```python
from build123d import *

# Parameters (mm, degrees)
BOSS_EXTRUDE1_DEPTH = 85
BOSS_EXTRUDE3_DEPTH = 2
SKETCH9_W           = 11.5
SKETCH9_H           = 2
BOSS_EXTRUDE8_DEPTH = 3
CHAMFER1_SIZE       = 3
SKETCH10_W          = 32
SKETCH10_H          = 85
BOSS_EXTRUDE9_DEPTH = 2
SKETCH11_W          = 15
SKETCH11_H          = 5
CUT_EXTRUDE1_DEPTH  = 108.588010242


with BuildPart() as part:
    # Sketch1 → Boss-Extrude1 (new body)
    with BuildSketch(Plane(origin=(0, 0, 0), x_dir=(1, 0, 0), z_dir=(0, 1, 0))):
        with BuildLine():
            Line((-29, -15), (-29, 15.762564303))
            ThreePointArc((-29, 15.762564303), (0, 25.341269657), (29, 15.762564303))
            Line((29, 15.762564303), (29, -15))
            Line((29, -15), (29, -17))
            Line((29, -17), (27.5, -17))
            Line((27.5, -17), (16, -17))
            Line((16, -17), (16, -15))
            Line((16, -15), (27.5, -15))
            Line((27.5, -15), (27.5, 15))
            ThreePointArc((27.5, 15), (0, 23.841269657), (-27.5, 15))
            Line((-27.5, 15), (-27.5, -15))
            Line((-27.5, -15), (-16, -15))
            Line((-16, -15), (-16, -17))
            Line((-16, -17), (-27.5, -17))
            Line((-27.5, -17), (-29, -17))
            Line((-29, -17), (-29, -15))
        make_face()
    extrude(amount=BOSS_EXTRUDE1_DEPTH)

    # Sketch3 → Boss-Extrude3 (add)
    with BuildSketch(Plane(origin=(0, 85, 0), x_dir=(1, 0, 0), z_dir=(0, 1, 0))):
        with BuildLine():
            Line((-16, -17), (16, -17))
            Line((16, -17), (29, -17))
            Line((29, -17), (29, 15.762564303))
            ThreePointArc((29, 15.762564303), (0, 25.341269657), (-29, 15.762564303))
            Line((-29, 15.762564303), (-29, -17))
            Line((-29, -17), (-16, -17))
        make_face()
    extrude(amount=BOSS_EXTRUDE3_DEPTH)

    # Sketch9 → Boss-Extrude8 (add)
    with BuildSketch(Plane(origin=(0, 0, 15), x_dir=(-1, 0, 0), z_dir=(0, 0, -1))):
        with Locations((-21.75, 15)):
            Rectangle(SKETCH9_W, SKETCH9_H)
        with Locations((21.75, 15)):
            Rectangle(SKETCH9_W, SKETCH9_H)
    extrude(amount=BOSS_EXTRUDE8_DEPTH)

    # Chamfer1
    chamfer1_edges = [part.edges().sort_by_distance(p)[0] for p in [
        (-21.75, 14, 15),
        (21.75, 14, 15),
    ]]
    chamfer(chamfer1_edges, length=CHAMFER1_SIZE - 0.0001)  # a hair under: the kernel refuses the full size

    # Sketch10 → Boss-Extrude9 (add)
    with BuildSketch(Plane.XY.offset(17)):
        with Locations((0, 42.5)):
            Rectangle(SKETCH10_W, SKETCH10_H)
    extrude(amount=-BOSS_EXTRUDE9_DEPTH)

    # Sketch11 → Cut-Extrude1 (cut, through all)
    with BuildSketch(Plane(origin=(29, 0, 0), x_dir=(0, 0, -1), z_dir=(1, 0, 0))):
        with Locations((0, 7.985525628)):
            Rectangle(SKETCH11_W, SKETCH11_H)
    extrude(amount=-CUT_EXTRUDE1_DEPTH, mode=Mode.SUBTRACT)


solid = part.part
```
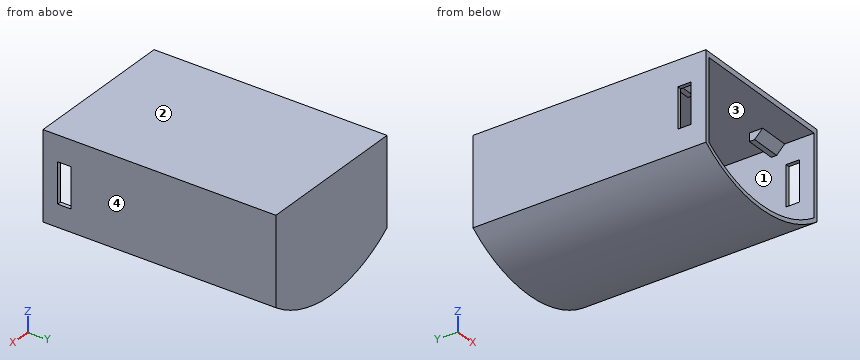
Work out the finished part from the listing and answer in its coordinate system (mm). Face numbers are marked on the shaded views. Round coordinates to 2 decimals unless told otherwise and drop trailing zeros. Write each loop counter-clockwise with the first axis right and the second up, starting at its lowest first coordinate (ties: lowest second). Pieces come first, ordered by that corner, then holes. Notation, with made-up numbers: (0, -2) -> (56, -2) arc R13 ccw to (56, 6) -> close; hole circle Ø3 at (-37.75, 48). An arc over 180 degrees is marked (long way). Write each question's results on one line, items separated by ' | '.
1) Consider line 1 along X through (y, z) = (70.5, 0); line 2 along Y through (x, z) = (-3, -7.5); line 3 along Z through (x, y) = (23, 14). Determine where each line is inside the solid, lowest interval first. Write a range as [from, to].
Findings:
line 1: x = [-29, -27.5], [27.5, 29] | line 2: y = [85, 87] | line 3: z = [-19.57, -17.86], [12, 17]
2) The part is cut by section D-D (z = -11). Write down the section's boundary in (x, y), and give its area (3 significant figures).
Findings:
outline: (-29, 0) -> (-27.5, 0) -> (-27.5, 85) -> (27.5, 85) -> (27.5, 0) -> (29, 0) -> (29, 87) -> (-29, 87) -> close | area: 371 mm²
3) Flat-ended cylindrical pins translate along their axes: pin 1 (1.2 mm diameter, centred on x = 28, y = 7, fed in from -Z); pin 2 (5 mm diameter, centred on x = -5, y = 66, fed in from -Z); pin 3 (8 mm diameter, centred on x = 23, y = 40, fed in from -Z). Find the tip coordinate at first contact, or state that the pin passes through.
Findings:
pin 1: stops at z = -16.9 | pin 2: stops at z = -25.28 | pin 3: stops at z = -21.48
4) The part is cut by section A-A (z = 3.5). Write down the section's boundary in (x, y), and give its area (3 significant figures).
Findings:
outline: (-29, 0) -> (-27.5, 0) -> (-27.5, 5.49) -> (-29, 5.49) -> close; (-29, 10.49) -> (-27.5, 10.49) -> (-27.5, 85) -> (27.5, 85) -> (27.5, 10.49) -> (29, 10.49) -> (29, 87) -> (-29, 87) -> close; (27.5, 0) -> (29, 0) -> (29, 5.49) -> (27.5, 5.49) -> close | area: 356 mm²
5) The part is cut by section B-B (y = 32). Write down the section's boundary in (x, z), and give its area (3 significant figures).
Findings:
outline: (-29, -15.76) arc R48.69 ccw to (29, -15.76) -> (29, 17) -> (-29, 17) -> close; hole (-27.5, -15) arc R47.19 ccw to (27.5, -15) -> (27.5, 15) -> (-27.5, 15) -> close | area: 298 mm²
6) For a pull along Z with two mould halves and no side action, classify the marked faces 1, 2, 3 and 4 as +Z half, -Z half, draft (parallel to the pull), parting line (faces both ways), or undercut.
Findings:
face 1: undercut | face 2: +Z half | face 3: undercut | face 4: draft
